Autodesk Inventor part; units mm, degrees
ref_plane "YZ Plane" through (0, 0, 0) normal (1, 0, 0) x (0, 1, 0)
ref_plane "XZ Plane" through (0, 0, 0) normal (0, 1, 0) x (-1, 0, 0)
ref_plane "XY Plane" through (0, 0, 0) normal (0, 0, 1) x (1, 0, 0)
sketch "Sketch1" plane through (0, 0, 0) normal (0, 1, 0) x (-1, 0, 0)
  circle A0 centre (0, 0) radius 49
  circle A1 centre (0, 0) radius 3
  circle A2 centre (0, 12.5) radius 2
  circle A3 centre (-12.5, 0) radius 2
  circle A4 centre (0, -12.5) radius 2
  circle A5 centre (12.5, 0) radius 2
  dimension "d0" = 98
  dimension "d1" = 6
  dimension "d6" = 12.5
  dimension "d9" = 360
  dimension "d11" = 4
extrude "Extrusion1" add sketch "Sketch1" along normal blind 3
sketch "Sketch2" plane through (0, 3, 0) normal (0, 1, 0) x (1, 0, 0)
  circle A0 centre (-43.75, 0) radius 1.25
  circle A1 centre (0, 0) radius 49 construction
  circle A2 centre (-23.75, 0) radius 1.25
  circle A3 centre (-32.6, -8.7351) radius 1.25
  line L0 (0, 0) -> (-22.9407, -6.147) construction
  line L1 (0, 0) -> (-23.75, 0) construction
  arc A4 (-23.75, 0) -> (-22.9407, -6.147) centre (5.6453, 0.7432) ccw construction
  line L2 (-22.9407, -6.147) -> (-32.6, -8.7351) construction
  point P0 (-49, 0)
  dimension "d14" = 2.5
  dimension "d16" = 5.25
  dimension "d17" = 20
  dimension "d24" = 15
  dimension "d25" = 10
extrude "Extrusion2" cut sketch "Sketch2" against normal through all
pattern_circular "Circular Pattern1" count 12 over 360 about axis through (0, 0, 0) along (0, 1, 0) of "Extrusion2"
sketch "Sketch3" plane through (0, 3, 0) normal (0, 1, 0) x (1, 0, 0)
  circle A0 centre (-43.75, 0) radius 1.25
  line L0 (0, 0) -> (-43.75, 0)
  circle A1 centre (-37.8886, -21.875) radius 1.25
  line L1 (-37.8886, -21.875) -> (0, 0) construction
  circle A2 centre (-32.6, 8.7351) radius 1.25
  circle A3 centre (0, 0) radius 3
  circle A4 centre (0, 0) radius 43.75
  circle A5 centre (-23.75, 0) radius 1.25
  circle A6 centre (0, 0) radius 23.75
  circle A7 centre (0, 0) radius 33.75
  circle A8 centre (-12.5, 0) radius 2
  circle A9 centre (0, 0) radius 12.5
  line L2 (0, 0) -> (-32.6, 8.7351) construction
  dimension "d28" = 10
  dimension "d29" = 10
  dimension "d30" = 11.25
  dimension "d23" = 30
  dimension "d31" = 15
equation "\"d25\" = 0.5 * d17"
Work out the finished part from the listing and answer in its coordinate system (mm). Give positions to 0.01 mm unless a question says otherwise; leave off trailing zeros. Loops run counter-clockwise (first coordinate to the right, second up) from the corner with the lowest first, then second, coordinate; pieces in that order, holes last. Notation, with made-up numbers: (-5, -10) -> (16, -10) arc R15 cw to (16, -2) -> close; hole circle Ø5 at (-23, 16.5). An arc over 180 degrees is marked (long way). One line per question, with ' | ' between items. Start each with the question number.
1) Section A-A, the plane x = 0 is taken. State how many separate pieces and enclosed holes the cut face has, then the cut area to 3 significant figures.
2) Section B-B, the plane x = -43.75 is taken. Determine the outline of the cut face in (y, z), then the cut area to 3 significant figures.
3) Straight lines are drawn through the part: L1, parallel to Z at x = -24.5, y = 0.8; L2, parallel to X at y = 0.85, z = -33; L3, parallel to Z at x = 9.5, y = 2.8. For each, find the intervals that lie inside material, in ascending order.
4) Determine the mould class of faces 1 (the face through (-10, 3, 1)), 2 (the face through (-23.702, 1.521, -22.626)) for opening direction Z: +Z half, -Z half, draft (parallel to the pull), parting line (faces both ways), or undercut.
5) Section C-C, the plane z = 43.75 is taken. Determine the outline of the cut face in (x, y).
Resolved:
1) separate pieces: 8 | enclosed holes: 0 | area: 222 mm2
2) outline: (0, -22.07) -> (3, -22.07) -> (3, -1.25) -> (0, -1.25) -> close; (0, 1.25) -> (3, 1.25) -> (3, 22.07) -> (0, 22.07) -> close | area: 125 mm2
3) L1: -42.44 to -24.94, -22.79 to -1, 1 to 22.79, 24.94 to 42.44 | L2: -36.22 to -9.92, -7.55 to 7.55, 9.92 to 36.22 | L3: -48.07 to -33.59, -31.61 to 31.61, 33.59 to 48.07
4) face 1: draft | face 2: undercut
5) outline: (-22.07, 0) -> (-1.25, 0) -> (-1.25, 3) -> (-22.07, 3) -> close; (1.25, 0) -> (22.07, 0) -> (22.07, 3) -> (1.25, 3) -> close
